CAD build for the part. Positions are in the model's coordinates, mm. Face numbers are marked on the shaded views. A direction names the side the tool comes from. Coordinates: 2 decimals unless noted, no trailing zeros. Loops run counter-clockwise (first coordinate to the right, second up) from the corner with the lowest first, then second, coordinate; pieces in that order, holes last. Notation, with made-up numbers: (-13.75, -22) -> (12.25, -22) arc R24 ccw to (12.25, -8) -> close; hole circle Ø7 at (-21.5, 17). An arc over 180 degrees is marked (long way). Write each question's results on one line, items separated by ' | '.
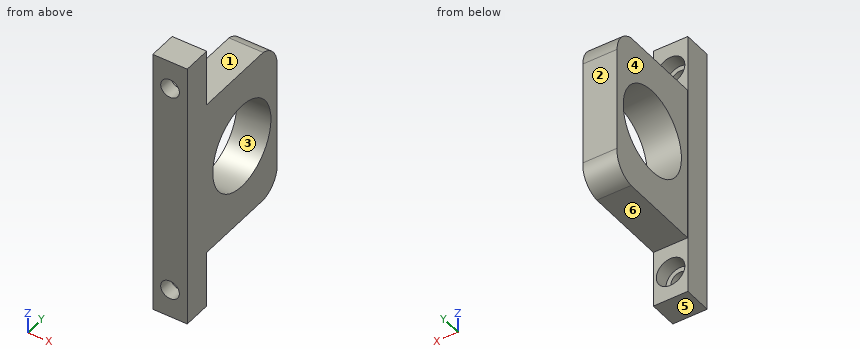
from build123d import *

# Parameters (mm, degrees)
SKETCH1_W           = 2.417978287
SKETCH1_H           = 19.01
SKETCH1_R           = 0.655
BOSS_EXTRUDE1_DEPTH = 2
SKETCH2_R           = 1
CUT_EXTRUDE1_DEPTH  = 1
SKETCH4_R           = 3
BOSS_EXTRUDE3_DEPTH = 2.4


with BuildPart() as part:
    # Sketch1 → Boss-Extrude1 (new body)
    with BuildSketch(Plane(origin=(0, 0, 0), x_dir=(1, 0, 0), z_dir=(0, 1, 0))):
        with Locations((-1.208989143, 14.330251099)):
            Rectangle(SKETCH1_W, SKETCH1_H)
        with Locations(Location((-1.207978287, 6.825251099, 0), (0, 0, 270))):
            Circle(SKETCH1_R, mode=Mode.SUBTRACT)
        with Locations(Location((-1.207978287, 21.835251099, 0), (0, 0, 270))):
            Circle(SKETCH1_R, mode=Mode.SUBTRACT)
    extrude(amount=BOSS_EXTRUDE1_DEPTH)

    # Sketch2 → Cut-Extrude1 (cut)
    with BuildSketch(Plane(origin=(0, 2, 0), x_dir=(1, 0, 0), z_dir=(0, 1, 0))):
        with Locations(Location((-1.207978287, 21.835251099, 0), (0, 0, 270))):
            Circle(SKETCH2_R)
        with Locations(Location((-1.207978287, 6.825251099, 0), (0, 0, 270))):
            Circle(SKETCH2_R)
    extrude(amount=-CUT_EXTRUDE1_DEPTH, mode=Mode.SUBTRACT)

    # Sketch4 → Boss-Extrude3 (add)
    with BuildSketch(Plane(origin=(0, 0, 0), x_dir=(0, 0, -1), z_dir=(1, 0, 0))):
        with BuildLine():
            Line((19.835251099, 2), (8.825251099, 2))
            Line((8.825251099, 2), (8.825251099, 7.833489784))
            ThreePointArc((8.825251099, 7.833489784), (9.485303513, 8.868997702), (10.645251099, 9.272070197))
            Line((10.645251099, 9.272070197), (18.019492282, 9.272070197))
            ThreePointArc((18.019492282, 9.272070197), (19.22631207, 8.930098925), (19.835251099, 7.833489784))
            Line((19.835251099, 7.833489784), (19.835251099, 2))
        make_face()
        with Locations((14.330251099, 5.636035099)):
            Circle(SKETCH4_R, mode=Mode.SUBTRACT)
    extrude(amount=-BOSS_EXTRUDE3_DEPTH)


solid = part.part
1) Two-plate mould, pull along Y, no slides. Class the marked faces 1, 2 and 3: pulls with the +Y half, pulls with the -Y half, needs draft (parallel to the pull), parting line crosses it, or undercut.
Outcome:
face 1: needs draft | face 2: pulls with the +Y half | face 3: undercut
2) Slice it at B-B (x = -1). Write the cut outline in (y, z), then the cut area to 3 significant figures.
Outcome:
outline: (0, -23.84) -> (2, -23.84) -> (2, -22.81) -> (1, -22.81) -> (1, -22.46) -> (0, -22.46) -> close; (0, -21.21) -> (1, -21.21) -> (1, -20.86) -> (2, -20.86) -> (2, -19.84) -> (7.83, -19.84) arc R1.63 ccw to (9.27, -18.02) -> (9.27, -10.65) arc R1.87 ccw to (7.83, -8.83) -> (2, -8.83) -> (2, -7.8) -> (1, -7.8) -> (1, -7.45) -> (0, -7.45) -> close; (0, -6.2) -> (1, -6.2) -> (1, -5.85) -> (2, -5.85) -> (2, -4.83) -> (0, -4.83) -> close; hole circle Ø6 at (5.64, -14.33) | area: 82.2 mm^2
3) Slice it at D-D (y = 1.5). Write the cut outline in (x, z), then the cut area to 3 significant figures.
Outcome:
outline: (-2.42, -23.84) -> (0, -23.84) -> (0, -4.83) -> (-2.42, -4.83) -> close; hole circle Ø2 at (-1.21, -21.84); hole circle Ø2 at (-1.21, -6.83) | area: 39.7 mm^2
4) Drill centre lines: L1, parallel to Z at x = -0.7, y = 5.5; L2, parallel to X at y = 0.5, z = -22.25; L3, parallel to X at y = 7, z = -19.5. Where is each one in solid material? Low to high. Write a range as from..to.
Outcome:
L1: z = -19.84..-17.33, -11.33..-8.83 | L2: x = -2.42..-1.71, -0.7..0 | L3: x = -2.4..0
5) Slice it at A-A (y = 6.75). Write the cut outline in (x, z), then the cut area to 3 significant figures.
Outcome:
outline: (-2.4, -19.84) -> (0, -19.84) -> (0, -17.12) -> (-2.4, -17.12) -> close; (-2.4, -11.54) -> (0, -11.54) -> (0, -8.83) -> (-2.4, -8.83) -> close | area: 13.1 mm^2
6) Pin check, flat tips, straight feed: pin 1 (0.7 mm diameter, centred on x = -1, y = 5, fed in from -Z); pin 2 (4 mm diameter, centred on y = 7.5, z = -11.5, fed in from -X); pin 3 (2 mm diameter, centred on y = 5, z = -14, fed in from -X); pin 4 (0.7 mm diameter, centred on x = -1, y = 4.5, fed in from +Z). Stop position of each tip, or through.
Outcome:
pin 1: stops at z = -19.84 | pin 2: stops at x = -2.4 | pin 3: passes through | pin 4: stops at z = -8.83
7) Which spindle directions (+Z, -Z, +X, -X, +Y, -Y) get a long thin tool onto all of the face, cutting with end or side? Do the marked faces 4, 5 and 6. Say none if no direction does.
Outcome:
face 4: +Z, -Z, -X, +Y | face 5: -Z, +X, -X, +Y, -Y | face 6: -Z, +X, -X, +Y
8) Slice it at C-C (z = -7). Write the cut outline in (x, y), then the cut area to 3 significant figures.
Outcome:
outline: (-2.42, 0) -> (-1.84, 0) -> (-1.84, 1) -> (-2.19, 1) -> (-2.19, 2) -> (-2.42, 2) -> close; (-0.58, 0) -> (0, 0) -> (0, 2) -> (-0.22, 2) -> (-0.22, 1) -> (-0.58, 1) -> close | area: 1.60 mm^2
